from build123d import *

# Parameters (mm, degrees)
SKETCH1_R      = 32.6
EXTRUDE1_DEPTH = 1


with BuildPart() as part:
    # Sketch1 → Extrude1 (new body)
    with BuildSketch(Plane(origin=(0, 0, 0), x_dir=(1, 0, 0), z_dir=(0, 1, 0))):
        Circle(SKETCH1_R)
        with BuildLine():
            Line((-7.5, 26.6), (-7.5, 21.319240137))
            ThreePointArc((-7.5, 21.319240137), (0, -22.6), (7.5, 21.319240137))
            Line((7.5, 21.319240137), (7.5, 26.6))
            Line((7.5, 26.6), (-7.5, 26.6))
        make_face(mode=Mode.SUBTRACT)
    extrude(amount=EXTRUDE1_DEPTH)


solid = part.part
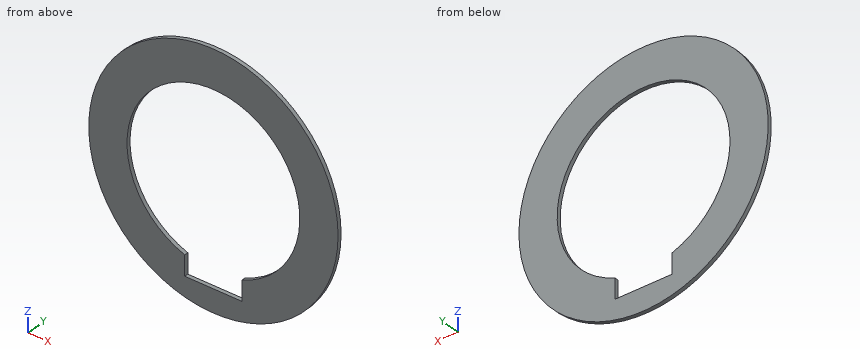
Build history of the part. All positions in model axes, mm. Round coordinates to 2 decimals unless told otherwise and drop trailing zeros. Write each loop counter-clockwise with the first axis right and the second up, starting at its lowest first coordinate (ties: lowest second). Pieces come first, ordered by that corner, then holes. Notation, with made-up numbers: M 43,46.25 L 89,46.25 A24 ccw 89,67.25 Z; hole C 74.5,-8 d10. An arc over 180 degrees is marked long. Use CSV: the item, a comma, the result in double quotes.
1. Wall check: probe 1 along X at (y, z) = (0.35, 0); probe 2 along Z at (x, y) = (0, 0.75); probe 3 along X at (y, z) = (0.2, -4). Give the ranges that are in metal, low to high. Write a range as from..to.
Reply:
probe 1,"x = -32.6..-22.6, 22.6..32.6"
probe 2,"z = -32.6..-26.6, 22.6..32.6"
probe 3,"x = -32.35..-22.24, 22.24..32.35"
2. Saw through at D-D (z = 24.5). Give the cut face in (x, y), plus the area to 3 significant figures.
Reply:
outline,"M -21.51,0 L 21.51,0 L 21.51,1 L -21.51,1 Z"
area,"43.0 mm²"
3. Saw through at A-A (x = 0). Give the cut face in (y, z), plus the area to 3 significant figures.
Reply:
outline,"M 0,-32.6 L 1,-32.6 L 1,-26.6 L 0,-26.6 Z; M 0,22.6 L 1,22.6 L 1,32.6 L 0,32.6 Z"
area,"16.0 mm²"
4. Flat gauge pins, fed straight in: pin 1 (6 mm diameter, centred on x = -14.5, z = -23.5, fed in from -Y); pin 2 (0.5 mm diameter, centred on y = 0.5, z = -23, fed in from +X). Where does each tip first touch, or does it go through?
Reply:
pin 1,"stops at y = 0"
pin 2,"stops at x = 23.35"
5. Saw through at B-B (z = 0). Give the cut face in (x, y), plus the area to 3 significant figures.
Reply:
outline,"M -32.6,0 L -22.6,0 L -22.6,1 L -32.6,1 Z; M 22.6,0 L 32.6,0 L 32.6,1 L 22.6,1 Z"
area,"20.0 mm²"
6. Saw through at C-C (y = 0.65). Give the cut face in (x, z), plus the area to 3 significant figures.
Reply:
outline,"C 0,0 d65.2; hole M -7.5,-26.6 L 7.5,-26.6 L 7.5,-21.32 A22.6 ccw long -7.5,-21.32 Z"
area,"1,670 mm²"
